```python
from build123d import *

# Parameters (mm, degrees)
SKETCH1_W           = 35
SKETCH1_H           = 16
SKETCH1_W_2         = 5
BOSS_EXTRUDE1_DEPTH = 6
SKETCH1_4_W         = 5
SKETCH1_4_H         = 16
BOSS_EXTRUDE2_DEPTH = 14
SKETCH4_R           = 2.5
CUT_EXTRUDE1_DEPTH  = 14
SKETCH3_R           = 1.25
CUT_EXTRUDE2_DEPTH  = 14
FILLET1_R           = 0.7
CUT_EXTRUDE3_DEPTH  = 3


with BuildPart() as part:
    # Sketch1 → Boss-Extrude1 (new body)
    with BuildSketch(Plane(origin=(0, 0, 0), x_dir=(1, 0, 0), z_dir=(0, 1, 0))):
        with Locations((17.5, 8)):
            Rectangle(SKETCH1_W, SKETCH1_H)
        with Locations((37.5, 8)):
            Rectangle(SKETCH1_W_2, SKETCH1_H)
    extrude(amount=BOSS_EXTRUDE1_DEPTH)

    # Sketch1_4 → Boss-Extrude2 (add)
    with BuildSketch(Plane(origin=(0, 0, 0), x_dir=(1, 0, 0), z_dir=(0, 1, 0))):
        with Locations((37.5, 8)):
            Rectangle(SKETCH1_4_W, SKETCH1_4_H)
    extrude(amount=BOSS_EXTRUDE2_DEPTH)

    # Sketch4 → Cut-Extrude1 (cut)
    with BuildSketch(Plane(origin=(0, 6, 0), x_dir=(1, 0, 0), z_dir=(0, 1, 0))):
        with Locations(Location((21, 8, 0), (0, 0, 270))):
            Circle(SKETCH4_R)
        with Locations(Location((6, 8, 0), (0, 0, 270))):
            Circle(SKETCH4_R)
    extrude(amount=-CUT_EXTRUDE1_DEPTH, mode=Mode.SUBTRACT)

    # Sketch3 → Cut-Extrude2 (cut)
    with BuildSketch(Plane.ZY.offset(-35)):
        with Locations((-13, 10)):
            Circle(SKETCH3_R)
        with Locations((-3, 10)):
            Circle(SKETCH3_R)
    extrude(amount=-CUT_EXTRUDE2_DEPTH, mode=Mode.SUBTRACT)

    # Fillet1
    fillet1_edges = [part.edges().sort_by_distance(p)[0] for p in [
        (40, 7, -16),
        (40, 7, 0),
        (35, 10, -16),
        (35, 10, 0),
        (0, 3, 0),
        (0, 3, -16),
    ]]
    fillet(fillet1_edges, radius=FILLET1_R)

    # Sketch5 → Cut-Extrude3 (cut)
    with BuildSketch(Plane.ZY.offset(-35)):
        Polygon((-11.556624327, 12.5), (-14.443375673, 12.5), (-15.886751346, 10), (-14.443375673, 7.5), (-11.556624327, 7.5), (-10.113248654, 10), align=None)
        Polygon((-4.443375673, 12.5), (-5.886751346, 10), (-4.443375673, 7.5), (-1.556624327, 7.5), (-0.113248654, 10), (-1.556624327, 12.5), align=None)
    extrude(amount=-CUT_EXTRUDE3_DEPTH, mode=Mode.SUBTRACT)


solid = part.part
```
Can you work these out from the model? Positions are in its coordinate system, mm. A direction names the side the tool comes from. Coordinates: 2 decimals unless noted, no trailing zeros. Loops run counter-clockwise (first coordinate to the right, second up) from the corner with the lowest first, then second, coordinate; pieces in that order, holes last. Notation, with made-up numbers: M -30,6 L 0,6 A9 cw 0,18 Z; hole C -35,16.5 d8. An arc over 180 degrees is marked long. Put each result on its own line as item: value. Start each with the question number.
(1) Imagine slicing it at A-A on z = -13. List the corners of the cut face in (x, y) for me, and give its area (3 significant figures).
(2) Imagine slicing it at C-C on z = -6.5. List the corners of the cut face in (x, y) for me.
(3) We'd pull the mould along Z, two halves only. Please class faces 4 (the face through (36, 12.5, -13)), 5 (the face through (37, 14, -8)), 6 (the face through (20, 4, 0)): +Z half, -Z half, draft (parallel to the pull), parting line (faces both ways), or undercut.
(4) I need wall thicknesses on probe 1 along X at (y, z) = (3.7, -8); probe 2 along Y at (x, z) = (39, -3); probe 3 along Y at (x, z) = (12, -8.25). Which ranges of each line are inside material? Lowest first, please.
(5) Which directions (+Z, -Z, +X, -X, +Y, -Y) give clear straight access to the entire face, cutting with the end or side of a thin tool? Please do faces 1 (the face through (35, 10, -8)), 2 (the face through (23.48, 3.04, -8.33)), 3 (the face through (36.479, 8.768, -15.175)).
(6) Will these pins go through, and if not, where does the flat tip stop? pin 1 Ø4 at (y, z) = (11.5, -11) entering from -X; pin 2 Ø2.5 at (y, z) = (10.5, -3.5) entering from -X.
(7) Imagine slicing it at D-D on x = 36.5. List the corners of the cut face in (y, z) for me, and give its area (3 significant figures).
(8) Imagine slicing it at B-B on x = 23. List the corners of the cut face in (y, z) for me.
Worked answers:
1. outline: M 0,0 L 40,0 L 40,8.75 L 38,8.75 L 38,7.5 L 35,7.5 L 35,6 L 0,6 Z; M 35,12.5 L 38,12.5 L 38,11.25 L 40,11.25 L 40,14 L 35,14 Z
1. area: 260 mm2
2. outline: M 0,0 L 4,0 L 4,6 L 0,6 Z; M 8,0 L 19,0 L 19,6 L 8,6 Z; M 23,0 L 40,0 L 40,14 L 35,14 L 35,6 L 23,6 Z
3. face 4: undercut
3. face 5: draft
3. face 6: +Z half
4. probe 1: x = 0 to 3.5, 8.5 to 18.5, 23.5 to 40
4. probe 2: y = 0 to 8.75, 11.25 to 14
4. probe 3: y = 0 to 6
5. face 1: +Z, -Z, -X, +Y
5. face 2: +Y, -Y
5. face 3: -X
6. pin 1: stops at x = 35
6. pin 2: stops at x = 38
7. outline: M 0,-16 L 14,-16 L 14,0 L 0,0 Z; hole M 7.5,-14.44 L 10,-15.89 L 12.5,-14.44 L 12.5,-11.56 L 10,-10.11 L 7.5,-11.56 Z; hole M 7.5,-4.44 L 10,-5.89 L 12.5,-4.44 L 12.5,-1.56 L 10,-0.11 L 7.5,-1.56 Z
7. area: 181 mm2
8. outline: M 0,-16 L 6,-16 L 6,-9.5 L 0,-9.5 Z; M 0,-6.5 L 6,-6.5 L 6,0 L 0,0 Z
